from build123d import *

# Parameters (mm, degrees)
F0_R     = 8
F0_R_2   = 5
F2_DEPTH = 18
F0_R_3   = 10
F3_DEPTH = 10
F4_START = 2
F0_R_4   = 11
F4_DEPTH = 6
F1_R     = 1.5
F5_DEPTH = 11.001
F6_R     = 1.5
F7_DEPTH = 11.001


with BuildPart() as f2:
    # F0 (on Top) → F2 (new body)
    with BuildSketch(Plane.XY):
        Circle(F0_R)
        Circle(F0_R_2, mode=Mode.SUBTRACT)
    extrude(amount=F2_DEPTH)

    # F0 (on Top) → F3 (join)
    with BuildSketch(Plane.XY):
        Circle(F0_R_3)
        Circle(F0_R, mode=Mode.SUBTRACT)
    extrude(amount=F3_DEPTH)

    # F0 (on Top) → F4 (join)
    with BuildSketch(Plane.XY.offset(F4_START)):
        Circle(F0_R_4)
        Circle(F0_R_3, mode=Mode.SUBTRACT)
    extrude(amount=F4_DEPTH)

    # F1 (on Right) → F5 (cut, through all)
    with BuildSketch(Plane.YZ):
        with Locations((0, 14)):
            Circle(F1_R)
    extrude(amount=F5_DEPTH, mode=Mode.SUBTRACT)

    # F6 (on Front) → F7 (cut, through all)
    with BuildSketch(Plane.XZ):
        with Locations((0, 14)):
            Circle(F6_R)
    extrude(amount=-F7_DEPTH, mode=Mode.SUBTRACT)


solid = f2.part
Build history of the part. All positions in model axes, mm. A direction names the side the tool comes from. Give positions to 0.01 mm unless a question says otherwise; leave off trailing zeros. Loops run counter-clockwise (first coordinate to the right, second up) from the corner with the lowest first, then second, coordinate; pieces in that order, holes last. Notation, with made-up numbers: (64.25, 88.5) - (123.25, 88.5) arc R31 ccw to (123.25, 115.5) - close; hole circle Ø4 at (11, -32.5). An arc over 180 degrees is marked (long way). Write item = value, one per line. Start each with the question number.
1) Tool access for faces 4 (the cylindrical face through (-1.73, -7.81, 13.94)), 5 (the cylindrical face through (-2.38, -10.74, 4.96)), 6 (the cylindrical face through (-2.17, -9.76, 0.99)), 7 (the cylindrical face through (-1.5, 6.36, 14.07)): list every direction of +Z, -Z, +X, -X, +Y, -Y with a clear straight run to the whole face (end or side of a thin tool).
2) Probe probe 1 along Y at (x, z) = (0, 8.25); probe 2 along Z at (x, y) = (0, 7.2); probe 3 along Z at (x, y) = (7, 6). List the from-to ranges inside material, lowest first. Write a range as from..to.
3) Pull direction Z, two halves, no side cores. Call faces 1 (the flat face through (5.2, 0.1, 18)), 2 (the flat face through (2, -10, 2)), 3 (the cylindrical face through (6.36, -1.5, 14.07)): +Z half, -Z half, draft (parallel to the pull), parting line (faces both ways), or undercut.
4) Band-saw the part on C-C on z = 14. Give the cut face in (x, y).
5) Drop flat-ended pins along their axis: pin 1 Ø2 at (y, z) = (-3.5, 6) entering from -X; pin 2 Ø2 at (x, z) = (5, 6) entering from -Y; pin 3 Ø4 at (y, z) = (0, 14) entering from -X. Give the stop position or say it passes through.
6) Band-saw the part on A-A on x = 0. Give the cut face in (y, z), plus the area to 3 significant figures.
7) Band-saw the part on D-D on y = -3.75. Give the cut face in (x, z), plus the area to 3 significant figures.
Final values:
q1.face_4 = +Z
q1.face_5 = +Z, -Z
q1.face_6 = -Z
q1.face_7 = +Y
q2.probe_1 = -10..-5, 5..10
q2.probe_2 = 0..12.5, 15.5..18
q2.probe_3 = 0..10
q3.face_1 = +Z half
q3.face_2 = -Z half
q3.face_3 = undercut
q4.outline = (-1.5, 4.77) - (-1.5, 7.86) arc R8 ccw (long way) to (7.86, -1.5) - (4.77, -1.5) arc R5 cw (long way) to start; (1.5, 4.77) arc R5 cw to (4.77, 1.5) - (7.86, 1.5) arc R8 ccw to (1.5, 7.86) - close
q5.pin_1 = -10.71
q5.pin_2 = -10.25
q5.pin_3 = -8
q6.outline = (-11, 2) - (-10, 2) - (-10, 0) - (-5, 0) - (-5, 18) - (-8, 18) - (-8, 10) - (-10, 10) - (-10, 8) - (-11, 8) - close; (5, 0) - (10, 0) - (10, 2) - (11, 2) - (11, 8) - (10, 8) - (10, 10) - (8, 10) - (8, 12.5) - (5, 12.5) - close; (5, 15.5) - (8, 15.5) - (8, 18) - (5, 18) - close
q6.area = 151 mm²
q7.outline = (-10.34, 2) - (-9.27, 2) - (-9.27, 0) - (-3.31, 0) - (-3.31, 18) - (-7.07, 18) - (-7.07, 10) - (-9.27, 10) - (-9.27, 8) - (-10.34, 8) - close; (3.31, 0) - (9.27, 0) - (9.27, 2) - (10.34, 2) - (10.34, 8) - (9.27, 8) - (9.27, 10) - (7.07, 10) - (7.07, 18) - (3.31, 18) - close
q7.area = 192 mm²
